```python
from build123d import *

# Parameters (mm, degrees)
SKETCH1_W             = 12.7
SKETCH1_H             = 3.175
BOSS_EXTRUDE1_DEPTH   = 203.2
M6_CLEARANCE_HOLE1_D  = 6.6
M5X0_8_TAPPED_HOLE1_D = 4.2
M6X1_0_TAPPED_HOLE1_D = 5
M5_CLEARANCE_HOLE1_D  = 5.5
M4_CLEARANCE_HOLE1_D  = 4.5


with BuildPart() as part:
    # Sketch1 → Boss-Extrude1 (new body)
    with BuildSketch(Plane.XY):
        with Locations((6.35, 1.5875)):
            Rectangle(SKETCH1_W, SKETCH1_H)
    extrude(amount=BOSS_EXTRUDE1_DEPTH)

    # M6 Clearance Hole1 (through all)
    with Locations(Plane(origin=(0, 0, 0), x_dir=(-1, 0, 0), z_dir=(0, -1, 0))):
        with Locations((-6.35, -6.35), (-6.35, -25.4)):
            Hole(M6_CLEARANCE_HOLE1_D / 2)

    # M5x0.8 Tapped Hole1 (through all)
    with Locations(Plane(origin=(0, 0, 0), x_dir=(-1, 0, 0), z_dir=(0, -1, 0))):
        with Locations((-6.35, -139.7), (-6.35, -107.95)):
            Hole(M5X0_8_TAPPED_HOLE1_D / 2)

    # M6x1.0 Tapped Hole1 (through all)
    with Locations(Plane(origin=(0, 3.175, 0), x_dir=(1, 0, 0), z_dir=(0, 1, 0))):
        with Locations((6.506704553, -171.45)):
            Hole(M6X1_0_TAPPED_HOLE1_D / 2)

    # M5 Clearance Hole1 (through all)
    with Locations(Plane(origin=(0, 3.175, 0), x_dir=(1, 0, 0), z_dir=(0, 1, 0))):
        with Locations((6.35, -196.85)):
            Hole(M5_CLEARANCE_HOLE1_D / 2)

    # M4 Clearance Hole1 (through all)
    with Locations(Plane(origin=(0, 0, 0), x_dir=(-1, 0, 0), z_dir=(0, -1, 0))):
        with Locations((-9.525, -184.15)):
            Hole(M4_CLEARANCE_HOLE1_D / 2)


solid = part.part
```
For this review, take the finished solid that the model builds, in its own axes (mm). Give positions to 0.01 mm unless a question says otherwise; leave off trailing zeros. Loops run counter-clockwise (first coordinate to the right, second up) from the corner with the lowest first, then second, coordinate; pieces in that order, holes last. Notation, with made-up numbers: M 46,25.5 L 103,25.5 A19 ccw 103,30.5 Z; hole C 53,-9.5 d11. An arc over 180 degrees is marked long. One line per item, written item: value. Start each with the question number.
Q1. Draft analysis for pull direction Z (two halves, no side actions). For faces 1 (the face through (5.92, 1.61, 22.13)), 2 (the face through (6, 0, 100)), 3 (the face through (6, 2, 203.2)), 4 (the face through (6.077, 1.61, 105.868)), state which applies: released by +Z, released by -Z, zero draft, split by the parting line, or undercut.
Q2. Add section B-B (y = 0.7). Give the boundary of the cut face in (x, z) (3 decimals), and give its area (3 significant figures).
Q3. Add section C-C (z = 171.45). Give the boundary of the cut face in (x, y) (3 decimals), and give its area (3 significant figures).
Q4. Add section A-A (z = 196.85). Give the boundary of the cut face in (x, y) (3 decimals).
Q5. For L1, parallel to X at y = 2.45, z = 196.85; L2, parallel to X at y = 2.3, z = 184.15 (3 decimals); L3, parallel to Z at x = 9.25, y = 1.95, list the stretches that pass through material, from the lowest coordinate up.
Reply:
1. face 1: undercut
1. face 2: zero draft
1. face 3: released by +Z
1. face 4: undercut
2. outline: M 0,0 L 12.7,0 L 12.7,203.2 L 0,203.2 Z; hole C 6.35,6.35 d6.6; hole C 6.35,25.4 d6.6; hole C 6.35,196.85 d5.5; hole C 6.507,171.45 d5; hole C 6.35,107.95 d4.2; hole C 6.35,139.7 d4.2; hole C 9.525,184.15 d4.5
2. area: 2,430 mm²
3. outline: M 0,0 L 4.007,0 L 4.007,3.175 L 0,3.175 Z; M 9.007,0 L 12.7,0 L 12.7,3.175 L 9.007,3.175 Z
3. area: 24.4 mm²
4. outline: M 0,0 L 3.6,0 L 3.6,3.175 L 0,3.175 Z; M 9.1,0 L 12.7,0 L 12.7,3.175 L 9.1,3.175 Z
5. L1: 0 to 3.6, 9.1 to 12.7
5. L2: 0 to 7.275, 11.775 to 12.7
5. L3: 0 to 4.78, 7.92 to 23.83, 26.97 to 181.92, 186.38 to 203.2
